Can you work these out from the model? Positions are in its coordinate system, mm. Face numbers are marked on the shaded views. Give positions to 0.01 mm unless a question says otherwise; leave off trailing zeros. Loops run counter-clockwise (first coordinate to the right, second up) from the corner with the lowest first, then second, coordinate; pieces in that order, holes last. Notation, with made-up numbers: (82.25, 2) -> (128.25, 2) arc R17 cw to (128.25, 32) -> close; hole circle Ø1 at (-1.75, 17.25). An arc over 180 degrees is marked (long way). Use CSV: the item, a comma, the result in double quotes.
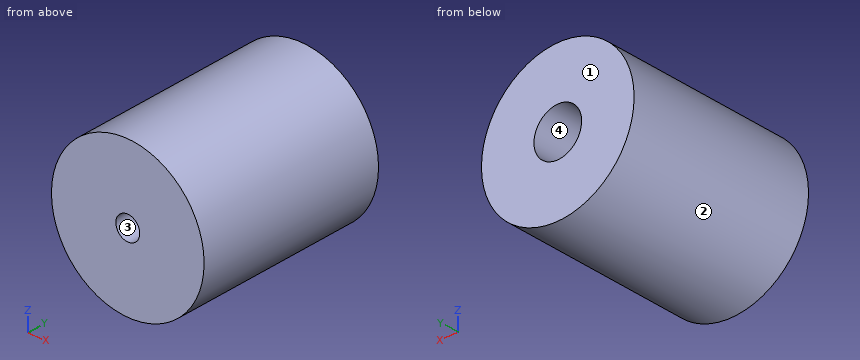
from build123d import *

# Parameters (mm, degrees)
SKETCH_1_R          = 6
EXTRUDE_1_DEPTH     = 40
SKETCH_2_R          = 5
CUT_EXTRUDE_2_DEPTH = 30
SKETCH_3_R          = 2.5
CUT_EXTRUDE_4_DEPTH = 10
SKETCH_5_R          = 16
SKETCH_5_R_2        = 6
EXTRUDE_1_2_DEPTH   = 40


with BuildPart() as part:
    # 草圖1 → Extrude 1 (new body)
    with BuildSketch(Plane(origin=(0, 0, 0), x_dir=(1, 0, 0), z_dir=(0, 1, 0))):
        with Locations(Location((0, 0, 0), (0, 0, 270))):
            Circle(SKETCH_1_R)
    extrude(amount=EXTRUDE_1_DEPTH)

    # 草圖2 → 除料-伸長2 (cut)
    with BuildSketch(Plane(origin=(0, 40, 0), x_dir=(1, 0, 0), z_dir=(0, 1, 0))):
        with Locations(Location((0, 0, 0), (0, 0, 270))):
            Circle(SKETCH_2_R)
    extrude(amount=-CUT_EXTRUDE_2_DEPTH, mode=Mode.SUBTRACT)

    # 草圖3 → 除料-伸長4 (cut)
    with BuildSketch(Plane.XZ):
        with Locations(Location((0, 0, 0), (0, 0, 270))):
            Circle(SKETCH_3_R)
    extrude(amount=-CUT_EXTRUDE_4_DEPTH, mode=Mode.SUBTRACT)

    # 草圖5 → Extrude 1 2 (add)
    with BuildSketch(Plane(origin=(0, 0, 0), x_dir=(1, 0, 0), z_dir=(0, 1, 0))):
        Circle(SKETCH_5_R)
        Circle(SKETCH_5_R_2, mode=Mode.SUBTRACT)
    extrude(amount=EXTRUDE_1_2_DEPTH)


solid = part.part
(1) If we section it at B-B, the plane z = 0: Write out the boundary of the cut face in (x, y).
Answer sheet:
outline,"(-16, 0) -> (-2.5, 0) -> (-2.5, 10) -> (-5, 10) -> (-5, 40) -> (-16, 40) -> close; (2.5, 0) -> (16, 0) -> (16, 40) -> (5, 40) -> (5, 10) -> (2.5, 10) -> close"
(2) If we section it at C-C, the plane y = 18: Write out the boundary of the cut face in (x, z), then the cut area to 3 significant figures.
Answer sheet:
outline,"circle Ø32 at (0, 0); hole circle Ø10 at (0, 0)"
area,"726 mm2"
(3) Will these pins go through, and if not, where does the flat tip stop? pin 1 Ø10 at (y, z) = (31, -11) entering from +X; pin 2 Ø1 at (x, y) = (-2, 17) entering from -Z; pin 3 Ø8 at (x, y) = (12.5, 28) entering from -Z.
Answer sheet:
pin 1,"stops at x = 14.83"
pin 2,"stops at z = -15.93"
pin 3,"stops at z = -13.56"
(4) If we section it at A-A, the plane x = 0: Write out the boundary of the cut face in (y, z), then the cut area to 3 significant figures.
Answer sheet:
outline,"(0, -16) -> (40, -16) -> (40, -5) -> (10, -5) -> (10, -2.5) -> (0, -2.5) -> close; (0, 2.5) -> (10, 2.5) -> (10, 5) -> (40, 5) -> (40, 16) -> (0, 16) -> close"
area,"930 mm2"
(5) We'd pull the mould along Z, two halves only. Please class the marked faces 1, 2, 3 and 4: released by +Z, released by -Z, zero draft, split by the parting line, or undercut.
Answer sheet:
face 1,"zero draft"
face 2,"split by the parting line"
face 3,"undercut"
face 4,"undercut"
(6) If we section it at D-D, the plane y = 3.5: Write out the boundary of the cut face in (x, z), then the cut area to 3 significant figures.
Answer sheet:
outline,"circle Ø32 at (0, 0); hole circle Ø5 at (0, 0)"
area,"785 mm2"
(7) If I drill on L1, parallel to X at y = 7.25, z = 0; L2, parallel to X at y = 27.5, z = 0; L3, parallel to X at y = 29, z = -9, over which ranges is the centre line in solid material (lowest first)? Write a range as from..to.
Answer sheet:
L1,"x = -16..-2.5, 2.5..16"
L2,"x = -16..-5, 5..16"
L3,"x = -13.23..13.23"
